Part model, mm, in its own coordinate system. Face numbers are marked on the shaded views. A direction names the side the tool comes from. Round coordinates to 2 decimals unless told otherwise and drop trailing zeros. Loops run counter-clockwise (first coordinate to the right, second up) from the corner with the lowest first, then second, coordinate; pieces in that order, holes last. Notation, with made-up numbers: M 33.25,-29.75 L 65.25,-29.75 A30 cw 65.25,-4.75 Z; hole C 3.25,45 d8. An arc over 180 degrees is marked long. Put each result on its own line as item: value. Start each with the question number.
1) Slice it at B-B on x = 0. Give the cut face in (y, z), then the cut area to 4 significant figures.
2) Probe line 1 along Y through (x, z) = (0, 2.35); line 2 along Z through (x, y) = (-6.5, -7.25); line 3 along Z through (x, y) = (-1.5, -9.5). List the from-to ranges inside material, lowest first.
3) Which spindle directions (+Z, -Z, +X, -X, +Y, -Y) get a long thin tool onto all of the face, cutting with end or side? Do the marked faces 1, 2 and 3. Say none if no direction does.
4) Slice it at D-D on x = 4.25. Give the cut face in (y, z).
5) Slice it at A-A on y = -7. Give the cut face in (x, z), then the cut area to 3 significant figures.
6) Slice it at C-C on y = -4.5. Give the cut face in (x, z).
7) Drop flat-ended pins along their axis: pin 1 Ø4.5 at (x, y) = (0, 6.869) entering from -Z; pin 2 Ø1.5 at (x, z) = (0, -2) entering from +Y; pin 3 Ø8 at (y, z) = (-3, -16) entering from +X; pin 4 Ø5 at (x, y) = (-0.5, -4.5) entering from +Z. Give the stop position or say it passes through.
8) Pull direction Y, two halves, no side cores. Call the marked faces 4, 5, 6 and 7: +Y half, -Y half, draft (parallel to the pull), parting line (faces both ways), or undercut.
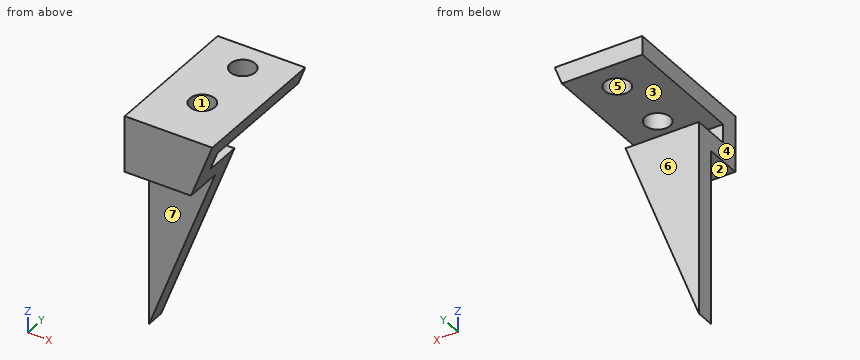
Autodesk Inventor part; units mm, degrees
ref_plane "YZ Plane" through (0, 0, 0) normal (1, 0, 0) x (0, 1, 0)
ref_plane "XZ Plane" through (0, 0, 0) normal (0, 1, 0) x (-1, 0, 0)
ref_plane "XY Plane" through (0, 0, 0) normal (0, 0, 1) x (1, 0, 0)
sketch "Эскиз1" plane through (0, 0, 0) normal (0, 0, 1) x (1, 0, 0)
  line L0 (-7, -11.5) -> (7, -11.5)
  line L1 (7, -11.5) -> (7, 11.5)
  line L2 (7, 11.5) -> (-7, 11.5)
  line L3 (-7, 11.5) -> (-7, -11.5)
  line L4 (-7, -11.5) -> (7, 11.5) construction
  line L5 (7, -11.5) -> (-7, 11.5) construction
  point P0 (0, 0)
  dimension "d0" = 14
  dimension "d1" = 23
extrude "Выдавливание1" add sketch "Эскиз1" along normal blind 3
sketch "Эскиз2" plane through (0, 0, 0) normal (0, 0, -1) x (-1, 0, 0)
  line L0 (7, -11.5) -> (-7, -11.5)
  line L1 (7, 11.5) -> (7, -11.5)
  line L2 (-7, 11.5) -> (7, 11.5)
  line L3 (-7, -11.5) -> (-7, 11.5)
  line L4 (7, -11.5) -> (7, -8.5)
  line L5 (7, 11.5) -> (7, -11.5) construction
  line L6 (7, -11.5) -> (-7, -11.5)
  line L7 (7, -8.5) -> (-7, -8.5)
  line L8 (-7, -8.5) -> (-7, -11.5)
  line L9 (-7, -11.5) -> (7, -11.5)
  line L10 (7, -11.5) -> (7, -8.5)
  point P0 (0, 0)
  dimension "d4" = 3
extrude "Выдавливание2" add sketch "Эскиз2" along normal blind 6 contours L0 L3 L7 L1
sketch "Эскиз3" plane through (-7, -8.5, 0) normal (0, 1, 0) x (1, 0, 0)
  line L0 (14, 6) -> (0, 6)
  line L1 (14, 0) -> (0, 0)
  line L2 (14, 0) -> (14, 6)
  line L3 (0, 6) -> (14, 6)
  line L4 (0, 0) -> (0, 6)
  line L5 (14, 6) -> (14, 3) construction
  line L6 (14, 0) -> (14, 6) construction
  line L7 (14, 3) -> (0, 3)
  line L8 (0, 3) -> (0, 6)
  line L9 (0, 6) -> (14, 6)
  line L10 (14, 6) -> (14, 3)
  point P0 (7, 0)
  dimension "d7" = 3
extrude "Выдавливание3" add sketch "Эскиз3" along normal blind 6 contours L2 L7 L4 L0
sketch "Эскиз4" plane through (0, 0, -6) normal (0, 0, -1) x (-1, 0, 0)
  line L0 (-7, -11.5) -> (7, -11.5)
  line L1 (7, -11.5) -> (7, -2.5)
  line L2 (-7, -2.5) -> (7, -2.5)
  line L3 (-7, -11.5) -> (-7, -2.5)
  line L4 (-7, -2.5) -> (7, -2.5) construction
  line L5 (-7, -2.5) -> (-7, -5.5) construction
  line L6 (-7, -5.5) -> (7, -5.5)
  line L7 (7, -5.5) -> (7, -2.5)
  line L8 (7, -2.5) -> (-7, -2.5)
  line L9 (-7, -2.5) -> (-7, -5.5)
  point P0 (0, 0)
  dimension "d10" = 3
extrude "Выдавливание4" add sketch "Эскиз4" along normal blind 28 contours L3 L2 L1 L6
sketch "Эскиз6" plane through (0, 0, 3) normal (0, 0, 1) x (1, 0, 0)
  line L0 (-7, -11.5) -> (7, -11.5)
  line L1 (7, -11.5) -> (7, 11.5)
  line L2 (7, 11.5) -> (-7, 11.5)
  line L3 (-7, 0) -> (7, 0) construction
  line L4 (7, -8.5) -> (7, 11.5) construction
  line L5 (7, 11.5) -> (-7, 11.5) construction
  line L6 (0, 11.5) -> (0, -11.5) construction
  line L7 (0, 0) -> (0, 11.5) construction
  line L8 (0, 5.75) -> (-7, 5.75) construction
  line L9 (-7, 10) -> (-7, -10) construction
  line L10 (0, 5.75) -> (7, 5.75) construction
  line L11 (0, -11.5) -> (0, 0) construction
  line L12 (0, -5.75) -> (7, -5.75) construction
  line L13 (-7, 11.5) -> (-7, -11.5)
  line L14 (0, -11.5) -> (0, -3.131) construction
  line L15 (0, -3.131) -> (0, 6.869) construction
  circle A0 centre (0, -3.131) radius 2
  circle A1 centre (0, 6.869) radius 2
  point P0 (-5.8649, 10)
  dimension "d21" = 8.369
  dimension "d22" = 10
  dimension "d23" = 4
  dimension "d24" = 4
extrude "Выдавливание6" cut sketch "Эскиз6" against normal up to next contours A0 | A1
sketch "Эскиз7" plane through (-7, -11.5, 3) normal (0, -1, 0) x (1, 0, 0)
  line L0 (14, -9) -> (14, 0)
  line L1 (0, 0) -> (14, 0)
  line L2 (0, 0) -> (0, -9)
  line L3 (14, -9) -> (0, -9)
  line L4 (0, -9) -> (14, -9)
  line L5 (0, -9) -> (0, -37)
  line L6 (14, -37) -> (0, -37)
  line L7 (14, -9) -> (14, -37)
  line L8 (0, 0) -> (14, 0)
  line L9 (0, -6) -> (0, -37)
  line L10 (14, 0) -> (0, -37)
  line L11 (0, -37) -> (14, -37)
  line L12 (14, -9) -> (14, 0)
  line L13 (14, 0) -> (14, -37)
  point P0 (7, -3)
extrude "Выдавливание7" cut sketch "Эскиз7" against normal blind 28 contours L3 L10 L0 | L7 L6 L10 L3
properties part number "Side control right"
Recorded:
1. outline: M -11.5,-6 L -5.5,-6 L -5.5,-15.5 L -2.5,-15.5 L -2.5,-3 L -8.5,-3 L -8.5,0 L -5.13,0 L -5.13,3 L -11.5,3 Z; M -1.13,0 L 4.87,0 L 4.87,3 L -1.13,3 Z; M 8.87,0 L 11.5,0 L 11.5,3 L 8.87,3 Z
1. area: 109.5 mm2
2. line 1: y = -11.5 to -5.13, -1.13 to 4.87, 8.87 to 11.5
2. line 2: z = -6 to -3, 0 to 3
2. line 3: z = -6 to 3
3. face 1: +Z
3. face 2: -Z, +X, -X, -Y
3. face 3: +X, -X, +Y
4. outline: M -11.5,-4.27 L -2.5,-4.27 L -2.5,-3 L -8.5,-3 L -8.5,0 L 11.5,0 L 11.5,3 L -11.5,3 Z
5. outline: M -7,-6 L 3.59,-6 L 4.73,-3 L -7,-3 Z; M -7,0 L 5.86,0 L 7,3 L -7,3 Z
5. area: 73.8 mm2
6. outline: M -7,-34 L 4.73,-3 L -7,-3 Z; M -7,0 L -1.46,0 L -1.46,3 L -7,3 Z; M 1.46,0 L 5.86,0 L 7,3 L 1.46,3 Z
7. pin 1: stops at z = 0
7. pin 2: stops at y = -8.5
7. pin 3: stops at x = 1.32
7. pin 4: stops at z = 3
8. face 4: draft
8. face 5: undercut
8. face 6: +Y half
8. face 7: -Y half
